from build123d import *

# Parameters (mm, degrees)
SKETCH1_W           = 27.5
SKETCH1_H           = 12.7
SKETCH1_R           = 1.5875
BOSS_EXTRUDE1_DEPTH = 6.35
FILLET1_R           = 1


with BuildPart() as part:
    # Sketch1 → Boss-Extrude1 (new body)
    with BuildSketch(Plane(origin=(0, 0, 0), x_dir=(1, 0, 0), z_dir=(0, 1, 0))):
        with Locations((13.75, 6.35)):
            Rectangle(SKETCH1_W, SKETCH1_H)
        with Locations((17.9125, 3.175)):
            Circle(SKETCH1_R, mode=Mode.SUBTRACT)
        Polygon((12.352283535, 3.175), (10.926141767, 5.64515), (8.073858233, 5.64515), (6.647716465, 3.175), (8.073858233, 0.70485), (10.926141767, 0.70485), align=None, mode=Mode.SUBTRACT)
    extrude(amount=BOSS_EXTRUDE1_DEPTH)

    # Fillet1
    fillet1_edges = [part.edges().sort_by_distance(p)[0] for p in [
        (0, 3.175, -12.7),
        (27.5, 3.175, -12.7),
        (27.5, 3.175, 0),
        (0, 3.175, 0),
    ]]
    fillet(fillet1_edges, radius=FILLET1_R)


solid = part.part
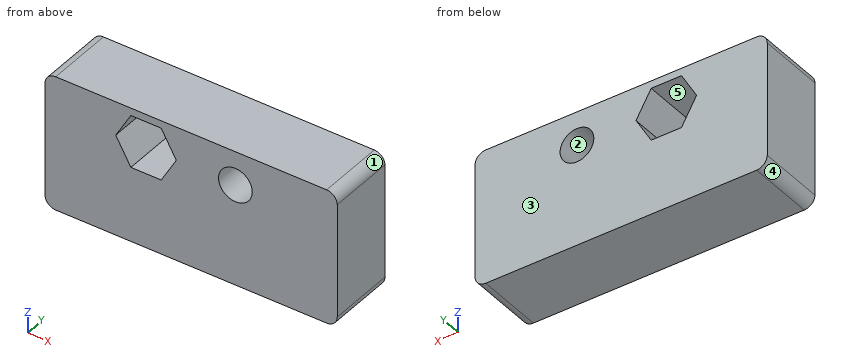
Could you check a few things on this model? Use its own coordinates, in mm. Face numbers are marked on the shaded views. A direction names the side the tool comes from. Round coordinates to 2 decimals unless told otherwise and drop trailing zeros. Write each loop counter-clockwise with the first axis right and the second up, starting at its lowest first coordinate (ties: lowest second). Pieces come first, ordered by that corner, then holes. Notation, with made-up numbers: (75.25, 52.5) -> (96.25, 52.5) arc R25 ccw to (96.25, 64.5) -> close; hole circle Ø2 at (16.5, -26.5). An arc over 180 degrees is marked (long way). Use a Markdown table: item, result.
1. We'd pull the mould along X, two halves only. Please class the marked faces 1, 2 and 3: +X half, -X half, draft (parallel to the pull), parting line (faces both ways), or undercut.
Answer key:
| item | result |
|---|---|
| face 1 | +X half |
| face 2 | undercut |
| face 3 | draft |
2. If we section it at C-C (x = 18.5): List the corners of the cut face in (y, z) for me.
Answer key:
| item | result |
|---|---|
| outline | (0, -12.7) -> (6.35, -12.7) -> (6.35, -4.65) -> (0, -4.65) -> close; (0, -1.7) -> (6.35, -1.7) -> (6.35, 0) -> (0, 0) -> close |
3. For pin 1 Ø1.9 at (x, z) = (17.91, -3.18) entering from -Y, with a flat end and sliding along its axis, tell me the tip position at first contact or that it passes through.
Answer key:
| item | result |
|---|---|
| pin 1 | passes through |
4. If we section it at B-B (z = -5.25): List the corners of the cut face in (x, y) for me, then the cut area to 3 significant figures.
Answer key:
| item | result |
|---|---|
| outline | (0, 0) -> (7.85, 0) -> (7.85, 6.35) -> (0, 6.35) -> close; (11.15, 0) -> (27.5, 0) -> (27.5, 6.35) -> (11.15, 6.35) -> close |
| area | 154 mm^2 |
5. Which directions (+Z, -Z, +X, -X, +Y, -Y) give clear straight access to the entire face, cutting with the end or side of a thin tool? Please do the marked faces 4 and 5.
Answer key:
| item | result |
|---|---|
| face 4 | -Z, -X, +Y, -Y |
| face 5 | +Y, -Y |
6. If we section it at A-A (y = 4.25): List the corners of the cut face in (x, z) for me (1 decimal).
Answer key:
| item | result |
|---|---|
| outline | (0, -11.7) arc R1 ccw to (1, -12.7) -> (26.5, -12.7) arc R1 ccw to (27.5, -11.7) -> (27.5, -1) arc R1 ccw to (26.5, 0) -> (1, 0) arc R1 ccw to (0, -1) -> close; hole (6.6, -3.2) -> (8.1, -5.6) -> (10.9, -5.6) -> (12.4, -3.2) -> (10.9, -0.7) -> (8.1, -0.7) -> close; hole circle Ø3.2 at (17.9, -3.2) |
7. Please list where these lines run through material, in increasing order: probe 1 along X at (y, z) = (3, -2.75); probe 2 along Z at (x, y) = (16.5, 3); probe 3 along X at (y, z) = (1, -2.25).
Answer key:
| item | result |
|---|---|
| probe 1 | x = 0 to 6.89, 12.11 to 16.38, 19.44 to 27.5 |
| probe 2 | z = -12.7 to -3.9, -2.45 to 0 |
| probe 3 | x = 0 to 7.18, 11.82 to 16.62, 19.2 to 27.5 |
